from build123d import *

# Parameters (mm, degrees)
SKETCH_1_R          = 2.5
EXTRUDE_4_DEPTH     = 2
SKETCH_4_R          = 1.5
CUT_EXTRUDE_2_DEPTH = 2
SKETCH_6_W          = 26.75
SKETCH_6_H          = 2
EXTRUDE_5_DEPTH     = 10
SKETCH_7_R          = 1.5
SKETCH_7_R_2        = 1.663234229
EXTRUDE_6_DEPTH     = 2
SKETCH_8_R          = 1.55
CUT_EXTRUDE_3_DEPTH = 2


with BuildPart() as part:
    # 草图1 → 凸台-拉伸4 (new body)
    with BuildSketch(Plane(origin=(0, 0, 0), x_dir=(1, 0, 0), z_dir=(0, 1, 0))):
        Polygon((0, 0), (0, -80), (70, -80), (100, -80), (100, 80), (70, 80), (0, 80), align=None)
        with Locations(Location((90, -50, 0), (0, 0, 270))):
            Circle(SKETCH_1_R, mode=Mode.SUBTRACT)
        with Locations(Location((90, 0, 0), (0, 0, 270))):
            Circle(SKETCH_1_R, mode=Mode.SUBTRACT)
        with Locations(Location((90, 50, 0), (0, 0, 270))):
            Circle(SKETCH_1_R, mode=Mode.SUBTRACT)
    extrude(amount=EXTRUDE_4_DEPTH)

    # 草图4 → 切除-拉伸2 (cut)
    with BuildSketch(Plane(origin=(0, 2, 0), x_dir=(1, 0, 0), z_dir=(0, 1, 0))):
        with BuildLine():
            Line((65.178018522, 50), (77.178018522, 50))
            ThreePointArc((77.178018522, 50), (80.006445646, 48.828427125), (81.178018522, 46))
            Line((81.178018522, 46), (81.178018522, -46))
            ThreePointArc((81.178018522, -46), (80.006445646, -48.828427125), (77.178018522, -50))
            Line((77.178018522, -50), (65.178018522, -50))
            ThreePointArc((65.178018522, -50), (62.349591397, -48.828427125), (61.178018522, -46))
            Line((61.178018522, -46), (61.178018522, 46))
            ThreePointArc((61.178018522, 46), (62.349591397, 48.828427125), (65.178018522, 50))
        make_face()
        with Locations(Location((47.4, -47.4, 0), (0, 0, 270))):
            Circle(SKETCH_4_R)
        with Locations(Location((47.4, 47.4, 0), (0, 0, 270))):
            Circle(SKETCH_4_R)
    extrude(amount=-CUT_EXTRUDE_2_DEPTH, mode=Mode.SUBTRACT)

    # 草图6 → 凸台-拉伸5 (add)
    with BuildSketch(Plane(origin=(0, 2, 0), x_dir=(1, 0, 0), z_dir=(0, 1, 0))):
        with Locations((13.375, -31.25)):
            Rectangle(SKETCH_6_W, SKETCH_6_H)
        with BuildLine():
            Line((47.25, 32.25), (46.75, 32.25))
            Line((46.75, 32.25), (46.75, 28.75))
            Line((46.75, 28.75), (46.75, -28.75))
            Line((46.75, -28.75), (46.75, -32.25))
            Line((46.75, -32.25), (47.25, -32.25))
            ThreePointArc((47.25, -32.25), (48.310660172, -31.810660172), (48.75, -30.75))
            Line((48.75, -30.75), (48.75, 30.75))
            ThreePointArc((48.75, 30.75), (48.310660172, 31.810660172), (47.25, 32.25))
        make_face()
        with BuildLine():
            Line((46.75, -32.25), (46.75, -28.75))
            ThreePointArc((46.75, -28.75), (46.310660172, -29.810660172), (45.25, -30.25))
            Line((45.25, -30.25), (45.25, -32.25))
            Line((45.25, -32.25), (46.75, -32.25))
        make_face()
        with BuildLine():
            Line((46.75, 32.25), (45.25, 32.25))
            Line((45.25, 32.25), (45.25, 30.25))
            ThreePointArc((45.25, 30.25), (46.310660172, 29.810660172), (46.75, 28.75))
            Line((46.75, 28.75), (46.75, 32.25))
        make_face()
        with Locations((13.375, 31.25)):
            Rectangle(SKETCH_6_W, SKETCH_6_H)
    extrude(amount=EXTRUDE_5_DEPTH)

    # 草图7 → 凸台-拉伸6 (add)
    with BuildSketch(Plane(origin=(0, 2, 0), x_dir=(1, 0, 0), z_dir=(0, 1, 0))):
        with Locations((47.4, 47.4)):
            Circle(SKETCH_7_R)
        with Locations((47.4, -47.4)):
            Circle(SKETCH_7_R_2)
    extrude(amount=-EXTRUDE_6_DEPTH)

    # 草图8 → 切除-拉伸3 (cut)
    with BuildSketch(Plane(origin=(0, 2, 0), x_dir=(1, 0, 0), z_dir=(0, 1, 0))):
        with BuildLine():
            ThreePointArc((47.95, 46.4), (47.496015511, 47.496015511), (46.4, 47.95))
            Line((46.4, 47.95), (46.4, 46.4))
            Line((46.4, 46.4), (47.95, 46.4))
        make_face()
        with BuildLine():
            Line((46.4, 46.4), (46.4, 47.95))
            ThreePointArc((46.4, 47.95), (45.303984489, 45.303984489), (47.95, 46.4))
            Line((47.95, 46.4), (46.4, 46.4))
        make_face()
        with Locations(Location((46.4, -46.4, 0), (0, 0, 270))):
            Circle(SKETCH_8_R)
    extrude(amount=-CUT_EXTRUDE_3_DEPTH, mode=Mode.SUBTRACT)


solid = part.part
Work out the finished part from the listing and answer in its coordinate system (mm). A direction names the side the tool comes from. Coordinates: 2 decimals unless noted, no trailing zeros. Write each loop counter-clockwise with the first axis right and the second up, starting at its lowest first coordinate (ties: lowest second). Pieces come first, ordered by that corner, then holes. Notation, with made-up numbers: M 21,-4.5 L 79,-4.5 A21 cw 79,34.5 Z; hole C -24,-23.75 d4. An arc over 180 degrees is marked long. Use one line per item in the form item = value. Start each with the question number.
1. The part is cut by section A-A (z = -9). Give the vertices of the cut face in (x, y).
2. Straight lines are drawn through the part: probe 1 along X at (y, z) = (1.35, 46.4); probe 2 along Z at (x, y) = (65.5, 1.25); probe 3 along Z at (x, y) = (5.5, 7.5). For each, find the intervals that lie inside material, in ascending order. Write a range as from..to.
3. Each of these flat-tipped pins is pushed along its axis until it touches: P1, Ø1.6, axis at x = 46.5, y = 5.5, coming from the +Z side; P2, Ø2, axis at y = 5, z = -31, coming from the +X side; P3, Ø4, axis at x = 46.4, z = -46.4, coming from the +Y side. Where does it stop, or does it pass through?
4. The part is cut by section D-D (z = -39.5). Give the vertices of the cut face in (x, y).
5. The part is cut by section B-B (x = 90). Give the vertices of the cut face in (y, z).
6. The mould has two halves that part along X. Classify faces 4 (the face through (62.38, 1.01, 48.86)), 5 (the face through (49, 0, -1)), 6 (the face through (48.75, 7, 0)): released by +X, released by -X, zero draft, split by the parting line, or undercut.
7. The part is cut by section C-C (x = 17.5). Give the vertices of the cut face in (y, z).
8. A tool of negligible diameter and unlimited length cuts with its end or side. For faces 1 (the face through (13, 7, 32.25)), 2 (the face through (80.037, 1.014, 48.797)), 3 (the face through (13, 7, 30.25)), from which of +Z, -Z, +X, -X, +Y, -Y can it reach the whole face along a straight path? Write none if from no direction.
Evaluation:
q1.outline = M 0,0 L 61.18,0 L 61.18,2 L 48.75,2 L 48.75,12 L 46.75,12 L 46.75,2 L 0,2 Z; M 81.18,0 L 100,0 L 100,2 L 81.18,2 Z
q2.probe_1 = 0..44.85, 47.95..61.2, 81.16..100
q2.probe_2 = -80..-50, 50..80
q2.probe_3 = -32.25..-30.25, 30.25..32.25
q3.P1 = 32.25
q3.P2 = 48.75
q3.P3 = 2
q4.outline = M 0,0 L 61.18,0 L 61.18,2 L 0,2 Z; M 81.18,0 L 100,0 L 100,2 L 81.18,2 Z
q5.outline = M 0,-80 L 2,-80 L 2,-52.5 L 0,-52.5 Z; M 0,-47.5 L 2,-47.5 L 2,-2.5 L 0,-2.5 Z; M 0,2.5 L 2,2.5 L 2,47.5 L 0,47.5 Z; M 0,52.5 L 2,52.5 L 2,80 L 0,80 Z
q6.face_4 = undercut
q6.face_5 = zero draft
q6.face_6 = released by +X
q7.outline = M 0,-80 L 2,-80 L 2,-32.25 L 12,-32.25 L 12,-30.25 L 2,-30.25 L 2,30.25 L 12,30.25 L 12,32.25 L 2,32.25 L 2,80 L 0,80 Z
q8.face_1 = +Z, +X, -X, +Y
q8.face_2 = +Y, -Y
q8.face_3 = -X, +Y
